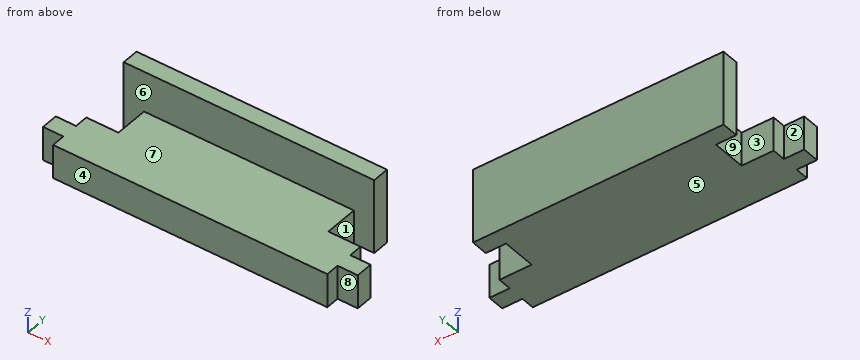
Autodesk Fusion 360 part; units mm, degrees
sketch "Sketch1" plane through (0, 0, 0) normal (0, 0, 1) x (1, 0, 0)
  line L0 (0, 0) -> (46.5, 0)
  line L1 (46.5, 0) -> (46.5, 15)
  line L2 (46.5, 15) -> (0, 15)
  line L3 (0, 15) -> (0, 0)
  dimension "d1" = 46.5
  dimension "d2" = 15
extrude "Extrude1" add sketch "Sketch1" along normal blind 11.5
sketch "Sketch2" plane through (0, 0, 11.5) normal (0, 0, 1) x (-1, 0, 0)
  line L0 (0, -15) -> (0, 0)
  line L1 (0, 0) -> (-46.5, 0)
  line L2 (-46.5, 0) -> (-46.5, -15)
  line L3 (-46.5, -15) -> (0, -15)
  line L4 (0, -15) -> (-4.75, -15)
  line L5 (-4.75, -15) -> (-4.75, -12.5)
  line L6 (-4.75, -12.5) -> (0, -12.5)
  line L7 (0, -12.5) -> (0, -15)
  dimension "d5" = 4.75
  dimension "d6" = 2.5
extrude "Extrude2" cut sketch "Sketch2" against normal blind 11.5 contours L0 L3 L4 L5 L6 L7
sketch "Sketch4" plane through (0, 0, 11.5) normal (0, 0, 1) x (-1, 0, 0)
  line L0 (-4.75, -12.5) -> (0, -12.5)
  line L1 (0, -12.5) -> (0, 0)
  line L2 (0, 0) -> (-46.5, 0)
  line L3 (-46.5, 0) -> (-46.5, -15)
  line L4 (-46.5, -15) -> (-4.75, -15)
  line L5 (-4.75, -15) -> (-4.75, -12.5)
  line L6 (-46.5, -15) -> (-41.75, -15)
  line L7 (-41.75, -15) -> (-41.75, -12.5)
  line L8 (-41.75, -12.5) -> (-46.5, -12.5)
  line L9 (-46.5, -12.5) -> (-46.5, -15)
  dimension "d11" = 4.75
  dimension "d12" = 2.5
extrude "Extrude3" cut sketch "Sketch4" against normal blind 11.5 contours L3 L4 L6 L7 L8 L9
sketch "Sketch5" plane through (0, 0, 11.5) normal (0, 0, 1) x (-1, 0, 0)
  line L0 (-41.75, -12.5) -> (-41.75, -15)
  line L1 (-41.75, -15) -> (-4.75, -15)
  line L2 (-4.75, -15) -> (-4.75, -12.5)
  line L3 (-4.75, -12.5) -> (0, -12.5)
  line L4 (0, -12.5) -> (0, 0)
  line L5 (0, 0) -> (-46.5, 0)
  line L6 (-46.5, 0) -> (-46.5, -12.5)
  line L7 (-46.5, -12.5) -> (-41.75, -12.5)
  line L8 (0, -12.5) -> (-4.75, -12.5)
  line L9 (-4.75, -12.5) -> (-4.75, -2.5)
  line L10 (-4.75, -2.5) -> (0, -2.5)
  line L11 (0, -2.5) -> (0, -12.5)
  dimension "d15" = 10
extrude "Extrude4" cut sketch "Sketch5" against normal blind 11.5 contours L3 L4 L8 L9 L10 L11
sketch "Sketch7" plane through (0, 0, 11.5) normal (0, 0, 1) x (-1, 0, 0)
  line L0 (-4.75, -2.5) -> (0, -2.5)
  line L1 (0, -2.5) -> (0, 0)
  line L2 (0, 0) -> (-46.5, 0)
  line L3 (-46.5, 0) -> (-46.5, -12.5)
  line L4 (-46.5, -12.5) -> (-41.75, -12.5)
  line L5 (-41.75, -12.5) -> (-41.75, -15)
  line L6 (-41.75, -15) -> (-4.75, -15)
  line L7 (-4.75, -15) -> (-4.75, -2.5)
  line L8 (-41.75, -12.5) -> (-46.5, -12.5)
  line L9 (-46.5, -12.5) -> (-46.5, -2.5)
  line L10 (-46.5, -2.5) -> (-41.75, -2.5)
  line L11 (-41.75, -2.5) -> (-41.75, -12.5)
  dimension "d18" = 10
extrude "Extrude5" cut sketch "Sketch7" against normal blind 11.5 contours L3 L4 L8 L9 L10 L11
sketch "Sketch8" plane through (0, 0, 11.5) normal (0, 0, 1) x (-1, 0, 0)
  line L0 (-41.75, -2.5) -> (-41.75, -15)
  line L1 (-41.75, -15) -> (-4.75, -15)
  line L2 (-4.75, -15) -> (-4.75, -2.5)
  line L3 (-4.75, -2.5) -> (0, -2.5)
  line L4 (0, -2.5) -> (0, 0)
  line L5 (0, 0) -> (-46.5, 0)
  line L6 (-46.5, 0) -> (-46.5, -2.5)
  line L7 (-46.5, -2.5) -> (-41.75, -2.5)
  line L8 (-4.75, -2.5) -> (-7.75, -2.5)
  line L9 (-7.75, -2.5) -> (-7.75, -12.5)
  line L10 (-7.75, -12.5) -> (-4.75, -12.5)
  line L11 (-4.75, -12.5) -> (-4.75, -2.5)
  dimension "d21" = 3
  dimension "d22" = 10
extrude "Extrude6" cut sketch "Sketch8" against normal blind 11.5 contours L2 L8 L9 L10 L11
sketch "Sketch9" plane through (0, 0, 11.5) normal (0, 0, 1) x (-1, 0, 0)
  line L0 (-4.75, -12.5) -> (-7.75, -12.5)
  line L1 (-7.75, -12.5) -> (-7.75, -2.5)
  line L2 (-7.75, -2.5) -> (0, -2.5)
  line L3 (0, -2.5) -> (0, 0)
  line L4 (0, 0) -> (-46.5, 0)
  line L5 (-46.5, 0) -> (-46.5, -2.5)
  line L6 (-46.5, -2.5) -> (-41.75, -2.5)
  line L7 (-41.75, -2.5) -> (-41.75, -15)
  line L8 (-41.75, -15) -> (-4.75, -15)
  line L9 (-4.75, -15) -> (-4.75, -12.5)
  line L10 (-41.75, -2.5) -> (-38.75, -2.5)
  line L11 (-38.75, -2.5) -> (-38.75, -12.5)
  line L12 (-38.75, -12.5) -> (-41.75, -12.5)
  line L13 (-41.75, -12.5) -> (-41.75, -2.5)
  dimension "d25" = 3
  dimension "d26" = 10
extrude "Extrude7" cut sketch "Sketch9" against normal blind 11.5 contours L7 L10 L11 L12 L13
sketch "Sketch10" plane through (0, 0, 11.5) normal (0, 0, 1) x (-1, 0, 0)
  line L0 (-46.5, -2.5) -> (-38.75, -2.5)
  line L1 (-38.75, -2.5) -> (-38.75, -12.5)
  line L2 (-38.75, -12.5) -> (-41.75, -12.5)
  line L3 (-41.75, -12.5) -> (-41.75, -15)
  line L4 (-41.75, -15) -> (-4.75, -15)
  line L5 (-4.75, -15) -> (-4.75, -12.5)
  line L6 (-4.75, -12.5) -> (-7.75, -12.5)
  line L7 (-7.75, -12.5) -> (-7.75, -2.5)
  line L8 (-7.75, -2.5) -> (0, -2.5)
  line L9 (0, -2.5) -> (0, 0)
  line L10 (0, 0) -> (-46.5, 0)
  line L11 (-46.5, 0) -> (-46.5, -2.5)
  line L12 (0, 0) -> (-46.5, 0)
  line L13 (-46.5, 0) -> (-46.5, -12.5)
  line L14 (-46.5, -12.5) -> (0, -12.5)
  line L15 (0, -12.5) -> (0, 0)
  dimension "d29" = 46.5
extrude "Extrude8" cut sketch "Sketch10" against normal blind 3.5 contours L0 L1 L7 L8 L9 L10 L11 L12 L13 L14 L15
sketch "Sketch11" plane through (0, 0, 0) normal (0, 0, -1) x (1, 0, 0)
  line L0 (38.75, -2.5) -> (46.5, -2.5)
  line L1 (46.5, -2.5) -> (46.5, 0)
  line L2 (46.5, 0) -> (0, 0)
  line L3 (0, 0) -> (0, -2.5)
  line L4 (0, -2.5) -> (7.75, -2.5)
  line L5 (7.75, -2.5) -> (7.75, -12.5)
  line L6 (7.75, -12.5) -> (4.75, -12.5)
  line L7 (4.75, -12.5) -> (4.75, -15)
  line L8 (4.75, -15) -> (41.75, -15)
  line L9 (41.75, -15) -> (41.75, -12.5)
  line L10 (41.75, -12.5) -> (38.75, -12.5)
  line L11 (38.75, -12.5) -> (38.75, -2.5)
  line L12 (0, 0) -> (46.5, 0)
  line L13 (46.5, 0) -> (46.5, -12.5)
  line L14 (46.5, -12.5) -> (0, -12.5)
  line L15 (0, -12.5) -> (0, 0)
  dimension "d32" = 46.5
  dimension "d33" = 12.5
extrude "Extrude9" cut sketch "Sketch11" against normal blind 3.5 contours L0 L1 L2 L3 L4 L5 L11 L12 L13 L14 L15
extrude "Extrude10" add 1 faces at (18.0833, 9.1667, 3.5) along direction (0, 0, -1) blind 3.5
extrude "Extrude11" cut 1 faces at (28.4167, 5.8333, 8) along direction (0, 0, -1) blind 3.5
extrude "Extrude12" add 1 faces at (18.0833, 12.5, 9.1667) along direction (0, -1, 0) blind 3
extrude "Extrude13" cut 1 faces at (29.4167, 15, 3.8333) along direction (0, -1, 0) blind 3
extrude "Extrude14" add 1 faces at (29.4167, 10.3333, 11.5) along direction (0, 0, 1) blind 1
extrude "Extrude15" add 1 faces at (17.0833, 12, 8.3333) along direction (0, 1, 0) blind 0.5
extrude "Extrude16" cut 1 faces at (17.0833, 11.5, 12.5) along direction (0, 0, -1) blind 0.5
extrude "Extrude17" add 1 faces at (31, 0, 3) along direction (0, -1, 0) blind 1
extrude "Extrude18" cut 1 faces at (31, -1, 3) along direction (0, 1, 0) blind 0.5
extrude "Extrude19" add 1 faces at (18.0833, 7.1667, 4.5) along direction (0, 0, 1) blind 0.5
sketch "Sketch12" plane through (38.75, 0, 0) normal (1, 0, 0) x (0, 1, 0)
  line L0 (9.5, 0) -> (9.5, 5)
  line L1 (9.5, 5) -> (2.5, 5)
  line L2 (2.5, 5) -> (2.5, 0)
  line L3 (2.5, 0) -> (9.5, 0)
  line L4 (2.5, 5) -> (4.5, 5)
  line L5 (4.5, 5) -> (4.5, 0)
  line L6 (4.5, 0) -> (2.5, 0)
  line L7 (2.5, 0) -> (2.5, 5)
  dimension "d56" = 2
extrude "Extrude20" add sketch "Sketch12" along normal blind 4.75 contours L1 L2 L3 L4 L5 L6 L7
sketch "Sketch13" plane through (7.75, 0, 0) normal (-1, 0, 0) x (0, -1, 0)
  line L0 (-9.5, 5) -> (-9.5, 0)
  line L1 (-9.5, 0) -> (-2.5, 0)
  line L2 (-2.5, 0) -> (-2.5, 5)
  line L3 (-2.5, 5) -> (-9.5, 5)
  line L4 (-2.5, 5) -> (-4.5, 5)
  line L5 (-4.5, 5) -> (-4.5, 0)
  line L6 (-4.5, 0) -> (-2.5, 0)
  line L7 (-2.5, 0) -> (-2.5, 5)
  dimension "d59" = 2
extrude "Extrude21" add sketch "Sketch13" along normal blind 4.75 contours L1 L2 L3 L4 L5 L6 L7
sketch "Sketch14" plane through (0, -0.5, 0) normal (0, -1, 0) x (1, 0, 0)
  line L0 (0, 5) -> (0, 0)
  line L1 (0, 0) -> (46.5, 0)
  line L2 (46.5, 0) -> (46.5, 5)
  line L3 (46.5, 5) -> (0, 5)
  line L4 (3, 0) -> (43.5, 0)
  line L5 (43.5, 0) -> (43.5, 5)
  line L6 (43.5, 5) -> (3, 5)
  line L7 (3, 5) -> (3, 0)
  dimension "d62" = 40.5
  dimension "d63" = 3
extrude "Extrude22" add sketch "Sketch14" along normal blind 2 contours L1 L3 L4 L5 L6 L7
extrude "Extrude23" cut 1 faces at (17.0833, 11.5, 12) along direction (0, 0, -1) blind 1
extrude "Extrude24" cut 1 faces at (29.4167, 12.5, 7.3333) along direction (0, -1, 0) blind 0.5
extrude "Extrude25" cut 1 faces at (45.5, -0.5, 3.3333) along direction (0, 1, 0) blind 0.5
extrude "Extrude26" cut 1 faces at (16.5, -2.5, 3.3333) along direction (0, 1, 0) blind 0.5
extrude "Extrude27" cut 1 faces at (1, -0.5, 3.3333) along direction (0, 1, 0) blind 0.5
The model under review builds one solid part; all positions refer to its coordinate system, in mm. Face numbers are marked on the shaded views. A direction names the side the tool comes from. Round coordinates to 2 decimals unless told otherwise and drop trailing zeros. Loops run counter-clockwise (first coordinate to the right, second up) from the corner with the lowest first, then second, coordinate; pieces in that order, holes last. Notation, with made-up numbers: M 22.5,62.25 L 36.5,62.25 A24 cw 36.5,92.25 Z; hole C 82,65 d6. An arc over 180 degrees is marked long. Answer as a JSON object with one key per item and string values.
Item 1: We need section C-C, the plane x = 12. State the section outline as (y, z) points.
Check sheet entries:
{"outline": "M -2,0 L 12,0 L 12,11 L 9.5,11 L 9.5,5 L -2,5 Z"}
Item 2: For line 1 along Y through (x, z) = (5.5, 4); line 2 along X through (y, z) = (3.75, 4.75); line 3 along X through (y, z) = (11, 7), list the stretches that pass through material, from the lowest coordinate up.
Check sheet entries:
{"line 1": "-2 to 4.5, 9.5 to 12", "line 2": "3 to 43.5", "line 3": "4.75 to 41.75"}
Item 3: We need section A-A, the plane x = 6. State the section outline as (y, z) points.
Check sheet entries:
{"outline": "M -2,0 L 4.5,0 L 4.5,5 L -2,5 Z; M 9.5,0 L 12,0 L 12,11 L 9.5,11 Z"}
Item 4: We need section D-D, the plane y = -0.5. State the section outline as (x, z) points.
Check sheet entries:
{"outline": "M 3,0 L 43.5,0 L 43.5,5 L 3,5 Z"}
Item 5: We need section B-B, the plane z = 4. State the section outline as (x, y) points.
Check sheet entries:
{"outline": "M 0,0 L 3,0 L 3,-2 L 43.5,-2 L 43.5,0 L 46.5,0 L 46.5,2.5 L 43.5,2.5 L 43.5,4.5 L 38.75,4.5 L 38.75,9.5 L 41.75,9.5 L 41.75,12 L 4.75,12 L 4.75,9.5 L 7.75,9.5 L 7.75,4.5 L 3,4.5 L 3,2.5 L 0,2.5 Z"}
Item 6: The part is to be moulded in two halves that separate along Y. For the marked faces 6, 7, 8 and 9, say which applies: +Y half, -Y half, draft (parallel to the pull), parting line (faces both ways), or undercut.
Check sheet entries:
{"face 6": "undercut", "face 7": "draft", "face 8": "-Y half", "face 9": "undercut"}
Item 7: Clearance check with flat-ended pins moving along their axes: P1, Ø4, axis at y = 8, z = 2, coming from the -X side; P2, Ø1, axis at y = -1.5, z = 3, coming from the -X side; P3, Ø3.5, axis at x = 32, z = 5.5, coming from the -Y side; P4, Ø0.8, axis at y = 10.5, z = 5.5, coming from the +X side. State where each tip first meets the part, or that it passes through.
Check sheet entries:
{"P1": "x = 4.75", "P2": "x = 3", "P3": "y = -2", "P4": "x = 41.75"}
Item 8: Tool access review of the marked faces 1, 2, 3, 4 and 5: name each direction out of +Z, -Z, +X, -X, +Y, -Y from which nothing blocks a thin tool from reaching the whole face with its end or side.
Check sheet entries:
{"face 1": "+Z, -Z, +X", "face 2": "+Z, -Z, -X, +Y", "face 3": "+Z, -Z, -X", "face 4": "+Z, -Z, +X, -X, -Y", "face 5": "-Z, +X, -X, +Y, -Y"}
